```python
from build123d import *

# Parameters (mm, degrees)
BOSS_EXTRUDE1_DEPTH = 20
SKETCH2_W           = 22
SKETCH2_H           = 14
CUT_EXTRUDE1_DEPTH  = 43.532340636
CUT_EXTRUDE2_DEPTH  = 45.362146026


with BuildPart() as part:
    # Sketch1 → Boss-Extrude1 (new body)
    with BuildSketch(Plane.XY):
        Polygon((0, 0), (0, 28), (3, 28), (3, 25), (25, 3), (28, 3), (28, 0), align=None)
    extrude(amount=BOSS_EXTRUDE1_DEPTH)

    # Sketch2 → Cut-Extrude1 (cut, through all)
    with BuildSketch(Plane(origin=(0, 3, 0), x_dir=(1, 0, 0), z_dir=(0, 1, 0))):
        with Locations((14, -10)):
            Rectangle(SKETCH2_W, SKETCH2_H)
    extrude(amount=CUT_EXTRUDE1_DEPTH, mode=Mode.SUBTRACT)

    # Sketch3 → Cut-Extrude2 (cut, through all)
    with BuildSketch(Plane.XZ):
        with BuildLine():
            Line((15.5, 6.75), (12.5, 6.75))
            ThreePointArc((12.5, 6.75), (9.25, 10), (12.5, 13.25))
            Line((12.5, 13.25), (15.5, 13.25))
            ThreePointArc((15.5, 13.25), (18.75, 10), (15.5, 6.75))
        make_face()
    cut_extrude2 = extrude(amount=-CUT_EXTRUDE2_DEPTH, mode=Mode.SUBTRACT)

    # Mirror1: Cut-Extrude2 across plane
    add(cut_extrude2.mirror(Plane(origin=(0, 0, 0), x_dir=(0, 0, 1), z_dir=(-0.7071067811865487, 0.7071067811865464, 0))), mode=Mode.SUBTRACT)


solid = part.part
```
Read the model definition and answer for the solid it produces. Units are mm, in the model's axes. A direction names the side the tool comes from. Coordinates: 2 decimals unless noted, no trailing zeros. Write each loop counter-clockwise with the first axis right and the second up, starting at its lowest first coordinate (ties: lowest second). Pieces come first, ordered by that corner, then holes. Notation, with made-up numbers: (26, -16.5) - (68, -16.5) arc R21 cw to (68, 18.5) - close; hole circle Ø1 at (67.25, -20). An arc over 180 degrees is marked (long way). Answer as a JSON object with one key per item and string values. Group by question number.
1. Consider L1, parallel to Z at x = 14.25, y = 7.25; L2, parallel to Y at x = 19.5, z = 8. Determine where each line is inside the solid, lowest interval first. Write a range as [from, to].
2. A cutting plane is placed at C-C (z = 17.5). Determine the outline of the cut face in (x, y).
3. Which of the six approach directions +Z, -Z, +X, -X, +Y, -Y give full straight-line access (tool end or side, diameter ignored) to faces 5 (the flat face through (14, 0, 5)), 6 (the flat face through (11, 11, 3)), 7 (the flat face through (1, 14, 13.25)), 8 (the flat face through (14, 1, 6.75))?
4. The mould has two halves that part along Y. Classify faces 1 (the flat face through (8, 8, 0)), 2 (the flat face through (18.1, 3, 7.6)), 3 (the flat face through (1, 14, 6.75)), 4 (the cylindrical face through (1.48, 18.75, 10.07)): +Y half, -Y half, draft (parallel to the pull), parting line (faces both ways), or undercut.
5. A cutting plane is placed at A-A (x = 14.25). Determine the outline of the cut face in (y, z).
6. A cutting plane is placed at B-B (y = 14.75). Determine the outline of the cut face in (x, z), plus the area to 3 significant figures.
7. Each of these flat-tipped pins is pushed along its axis until it touches: P1, Ø6, axis at x = 6.5, z = 4.5, coming from the +Y side; P2, Ø1.5, axis at x = 20, y = 10.5, coming from the +Z side; P3, Ø5, axis at y = 6.5, z = 4, coming from the +X side; P4, Ø6, axis at x = 21, z = 5.5, coming from the +Y side. Where does it stop, or does it pass through?
8. A cutting plane is placed at D-D (x = 4.75). Determine the outline of the cut face in (y, z), plus the area to 4 significant figures.
Worked out:
{
 "1": {"L1": "z = [0, 3], [17, 20]", "L2": "y = [0, 3]"},
 "2": {"outline": "(0, 0) - (28, 0) - (28, 3) - (25, 3) - (3, 25) - (3, 28) - (0, 28) - close"},
 "3": {"face 5": "+Z, -Z, +X, -X, -Y", "face 6": "+X, +Y", "face 7": "+X, -X", "face 8": "+Y, -Y"},
 "4": {"face 1": "draft", "face 2": "+Y half", "face 3": "undercut", "face 4": "undercut"},
 "5": {"outline": "(0, 0) - (13.75, 0) - (13.75, 3) - (3, 3) - (3, 6.75) - (0, 6.75) - close; (0, 13.25) - (3, 13.25) - (3, 17) - (13.75, 17) - (13.75, 20) - (0, 20) - close"},
 "6": {"outline": "(0, 0) - (13.25, 0) - (13.25, 3) - (3, 3) - (3, 6.75) - (0, 6.75) - close; (0, 13.25) - (3, 13.25) - (3, 17) - (13.25, 17) - (13.25, 20) - (0, 20) - close", "area": "102 mm²"},
 "7": {"P1": "stops at y = 24.1", "P2": "passes through", "P3": "stops at x = 23.79", "P4": "stops at y = 8.66"},
 "8": {"outline": "(0, 0) - (23.25, 0) - (23.25, 3) - (3, 3) - (3, 17) - (23.25, 17) - (23.25, 20) - (0, 20) - close", "area": "181.5 mm²"}
}
